from build123d import *


with BuildPart() as part:
    # Esquisse1 → Révolution1 (revolve)
    with BuildSketch(Plane.XY, mode=Mode.PRIVATE) as r_volution1_sk:
        with BuildLine():
            Line((98.182636899, 9.898736356), (98.182636899, 15.453384419))
            Line((98.182636899, 15.453384419), (101.558174274, 15.453384419))
            Line((101.558174274, 15.453384419), (101.558174274, 18.238189454))
            Line((101.558174274, 18.238189454), (112.461882094, 13.189244146))
            ThreePointArc((112.461882094, 13.189244146), (113.715718176, 12.094110728), (114.182636899, 10.496171735))
            Line((114.182636899, 10.496171735), (114.182636899, 6.689516504))
            ThreePointArc((114.182636899, 6.689516504), (113.743297071, 5.628856332), (112.682636899, 5.189516504))
            Line((112.682636899, 5.189516504), (110.916617784, 5.189516504))
            Line((110.916617784, 5.189516504), (110.916617784, 9.398736356))
            ThreePointArc((110.916617784, 9.398736356), (110.770171174, 9.752289746), (110.416617784, 9.898736356))
            Line((110.416617784, 9.898736356), (106.29719914, 9.898736356))
            ThreePointArc((106.29719914, 9.898736356), (103.00637414, 8.348852557), (99.715549141, 9.898736356))
            Line((99.715549141, 9.898736356), (98.182636899, 9.898736356))
        make_face()
    revolve(r_volution1_sk.sketch.rotate(Axis((81.048552149, 0, 0), (1, 0, 0)), 90), axis=Axis((81.048552149, 0, 0), (1, 0, 0)))


solid = part.part
Design review of the part built by this model. Coordinates are the model's own, in mm. A direction names the side the tool comes from. Give positions to 0.01 mm unless a question says otherwise; leave off trailing zeros. Loops run counter-clockwise (first coordinate to the right, second up) from the corner with the lowest first, then second, coordinate; pieces in that order, holes last. Notation, with made-up numbers: (-29, 88.5) - (18, 88.5) arc R20 ccw to (18, 96.5) - close; hole circle Ø4 at (-12.5, 15). An arc over 180 degrees is marked (long way). Use CSV: the item, a comma, the result in double quotes. Start each with the question number.
1. Insertion check: P1, Ø5, axis at x = 104, z = 0.5, coming from the +Y side; P2, Ø15, axis at y = -4, z = -1, coming from the -X side; P3, Ø2, axis at y = 10.5, z = -6, coming from the +X side; P4, Ø3, axis at x = 107.5, y = 7, coming from the -Z side. Each pin has a flat end and moves straight along its axis. Give the tip position at first contact, or say it passes through.
2. Draft analysis for pull direction Y (two halves, no side actions). For faces 4 (the cylindrical face through (98.938, 9.663, -2.146)), 5 (the flat face through (114.183, 7, 0)), 6 (the cylindrical face through (99.89, 13.71, 7.13)), state which applies: released by +Y, released by -Y, zero draft, split by the parting line, or undercut.
3. Add section C-C (x = 103.25). State the section outline as (y, z) points, plus the area to 3 significant figures.
4. Machinability: for faces 1 (the flat face through (101.558, -8, 14)), 2 (the flat face through (110.917, 4, -4)), 3 (the flat face through (98.183, 10.1, 0.2)), which of the approach directions +Z, -Z, +X, -X, +Y, -Y give a long, thin tool a straight path to every point of the face, cutting with its end or side? Answer none if there is none.
5. Add section A-A (z = 0). State the section outline as (x, y) points.
6. Wall thickness on L1, parallel to Y at x = 98.75, z = 0; L2, parallel to Z at x = 107.25, y = -3.5; L3, parallel to Z at x = 99, y = 4.5: over which ranges is each line inside the solid? List them lowest first.
Results found:
1,P1,"stops at y = 18.24"
1,P2,"stops at x = 98.18"
1,P3,"stops at x = 114.12"
1,P4,"stops at z = -14.84"
2,face 4,"undercut"
2,face 5,"zero draft"
2,face 6,"split by the parting line"
3,outline,"circle Ø34.91 at (0, 0); hole circle Ø16.71 at (0, 0)"
3,area,"738 mm²"
4,face 1,"-X"
4,face 2,"none"
4,face 3,"+Z, -Z, -X, +Y, -Y"
5,outline,"(98.18, -15.45) - (101.56, -15.45) - (101.56, -18.24) - (112.46, -13.19) arc R2.97 ccw to (114.18, -10.5) - (114.18, -6.69) arc R1.5 ccw to (112.68, -5.19) - (110.92, -5.19) - (110.92, -9.4) arc R0.5 cw to (110.42, -9.9) - (106.3, -9.9) arc R4.27 ccw to (99.72, -9.9) - (98.18, -9.9) - close; (98.18, 9.9) - (99.72, 9.9) arc R4.27 ccw to (106.3, 9.9) - (110.42, 9.9) arc R0.5 cw to (110.92, 9.4) - (110.92, 5.19) - (112.68, 5.19) arc R1.5 ccw to (114.18, 6.69) - (114.18, 10.5) arc R2.97 ccw to (112.46, 13.19) - (101.56, 18.24) - (101.56, 15.45) - (98.18, 15.45) - close"
6,L1,"y = -15.45 to -9.9, 9.9 to 15.45"
6,L2,"z = -15.2 to -9.26, 9.26 to 15.2"
6,L3,"z = -14.78 to -8.82, 8.82 to 14.78"
